Work out the finished part from the listing and answer in its coordinate system (mm). A direction names the side the tool comes from. Give positions to 0.01 mm unless a question says otherwise; leave off trailing zeros. Loops run counter-clockwise (first coordinate to the right, second up) from the corner with the lowest first, then second, coordinate; pieces in that order, holes last. Notation, with made-up numbers: (12, 0.25) - (38, 0.25) arc R6 ccw to (38, 6.25) - close; hole circle Ø9 at (12.25, 77.5). An arc over 180 degrees is marked (long way). One line per question, with ' | ' between items.
from build123d import *

# Parameters (mm, degrees)
CUT_EXTRUDE_START   = -6
CUT_EXTRUDE_1_DEPTH = 6


with BuildPart() as part:
    # 草图1 → 旋转1 (revolve)
    with BuildSketch(Plane.XY, mode=Mode.PRIVATE) as revolve_1_sk:
        Polygon((-59.358604437, 0), (-62.358604437, 0), (-62.358604437, 13.5), (-57.358604437, 13.5), (-57.358604437, 11.5), (-59.358604437, 11.5), (-59.358604437, 7), (-19.358604437, 7), (-19.358604437, 3.6), (-25.358604437, 3.6), (-25.358604437, 5.1), (-59.358604437, 5.1), align=None)
    revolve(revolve_1_sk.sketch.rotate(Axis((-81.741157905, 0, 0), (1, 0, 0)), 90), axis=Axis((-81.741157905, 0, 0), (1, 0, 0)))

    # 草图2 → 切除-拉伸1 (cut)
    with BuildSketch(Plane(origin=(-19.358604437, 0, 0), x_dir=(0, 0, -1), z_dir=(1, 0, 0)).offset(CUT_EXTRUDE_START)):
        with BuildLine():
            Line((-3.5, 3.709447398), (-3.5, -3.709447398))
            ThreePointArc((-3.5, -3.709447398), (0, -5.1), (3.5, -3.709447398))
            Line((3.5, -3.709447398), (3.5, 3.709447398))
            ThreePointArc((3.5, 3.709447398), (0, 5.1), (-3.5, 3.709447398))
        make_face()
    extrude(amount=CUT_EXTRUDE_1_DEPTH, mode=Mode.SUBTRACT)


solid = part.part
1. Find section A-A on y = 0. Write down the section's boundary in (x, z), then the cut area to 3 significant figures.
Evaluation:
outline: (-62.36, -13.5) - (-57.36, -13.5) - (-57.36, -11.5) - (-59.36, -11.5) - (-59.36, -7) - (-19.36, -7) - (-19.36, -3.6) - (-25.36, -3.6) - (-25.36, -5.1) - (-59.36, -5.1) - (-59.36, 5.1) - (-25.36, 5.1) - (-25.36, 3.6) - (-19.36, 3.6) - (-19.36, 7) - (-59.36, 7) - (-59.36, 11.5) - (-57.36, 11.5) - (-57.36, 13.5) - (-62.36, 13.5) - close | area: 259 mm2
2. Find section D-D on y = 8.25. Write down the section's boundary in (x, z).
Evaluation:
outline: (-62.36, -10.69) - (-57.36, -10.69) - (-57.36, -8.01) - (-59.36, -8.01) - (-59.36, 8.01) - (-57.36, 8.01) - (-57.36, 10.69) - (-62.36, 10.69) - close
3. Find section B-B on z = 0. Write down the section's boundary in (x, y).
Evaluation:
outline: (-62.36, -13.5) - (-57.36, -13.5) - (-57.36, -11.5) - (-59.36, -11.5) - (-59.36, -7) - (-19.36, -7) - (-19.36, -5.1) - (-59.36, -5.1) - (-59.36, 5.1) - (-19.36, 5.1) - (-19.36, 7) - (-59.36, 7) - (-59.36, 11.5) - (-57.36, 11.5) - (-57.36, 13.5) - (-62.36, 13.5) - close
4. Determine the mould class of faces 1 (the flat face through (-62.359, 0, 0)), 2 (the cylindrical face through (-59.82, 13.18, -2.93)), 3 (the flat face through (-22, -2, 3.5)) for opening direction Z: +Z half, -Z half, draft (parallel to the pull), parting line (faces both ways), or undercut.
Evaluation:
face 1: draft | face 2: parting line | face 3: undercut
5. Consider L1, parallel to Y at x = -57.95, z = 0; L2, parallel to X at y = -1.75, z = -4.5; L3, parallel to Y at x = -48, z = 0. Determine where each line is inside the solid, lowest interval first.
Evaluation:
L1: -13.5 to -11.5, -7 to -5.1, 5.1 to 7, 11.5 to 13.5 | L2: -62.36 to -59.36, -25.36 to -19.36 | L3: -7 to -5.1, 5.1 to 7
6. Flat-ended cylindrical pins translate along their axes: pin 1 (3 mm diameter, centred on x = -23.5, y = 3, fed in from -Z); pin 2 (8 mm diameter, centred on y = -10, z = -9.5, fed in from +X); pin 3 (3 mm diameter, centred on y = 2, z = -1, fed in from +X). Find the tip coordinate at first contact, or state that the pin passes through.
Evaluation:
pin 1: z = -6.84 | pin 2: x = -57.36 | pin 3: x = -59.36
7. Which of the six approach directions +Z, -Z, +X, -X, +Y, -Y give full straight-line access (tool end or side, diameter ignored) to faces 4 (the flat face through (-25.359, 0, 4)), 5 (the cylindrical face through (-22.4, 0, 3.6)), 6 (the flat face through (-19.359, 0, 5))?
Evaluation:
face 4: none | face 5: +X | face 6: +Z, -Z, +X, +Y, -Y
8. Find section C-C on x = -23. Write down the section's boundary in (y, z), then the cut area to 3 significant figures.
Evaluation:
outline: circle Ø14 at (0, 0); hole (-3.71, -3.5) - (-0.84, -3.5) arc R3.6 ccw to (0.84, -3.5) - (3.71, -3.5) arc R5.1 ccw to (3.71, 3.5) - (0.84, 3.5) arc R3.6 ccw to (-0.84, 3.5) - (-3.71, 3.5) arc R5.1 ccw to start | area: 88.4 mm2
